Can you work these out from the drawing? Everything is in mm from the part's minimum corner. A direction names the side the tool comes from. Coordinates: 2 decimals unless noted, no trailing zeros. Loops run counter-clockwise (first coordinate to the right, second up) from the corner with the lowest first, then second, coordinate; pieces in that order, holes last. Notation, with made-up numbers: (50.25, -39.75) -> (95.25, -39.75) arc R25 ccw to (95.25, -25.75) -> close; hole circle Ø6 at (-18, -26.5). An arc over 180 degrees is marked (long way). One line per question, with ' | ' between items.
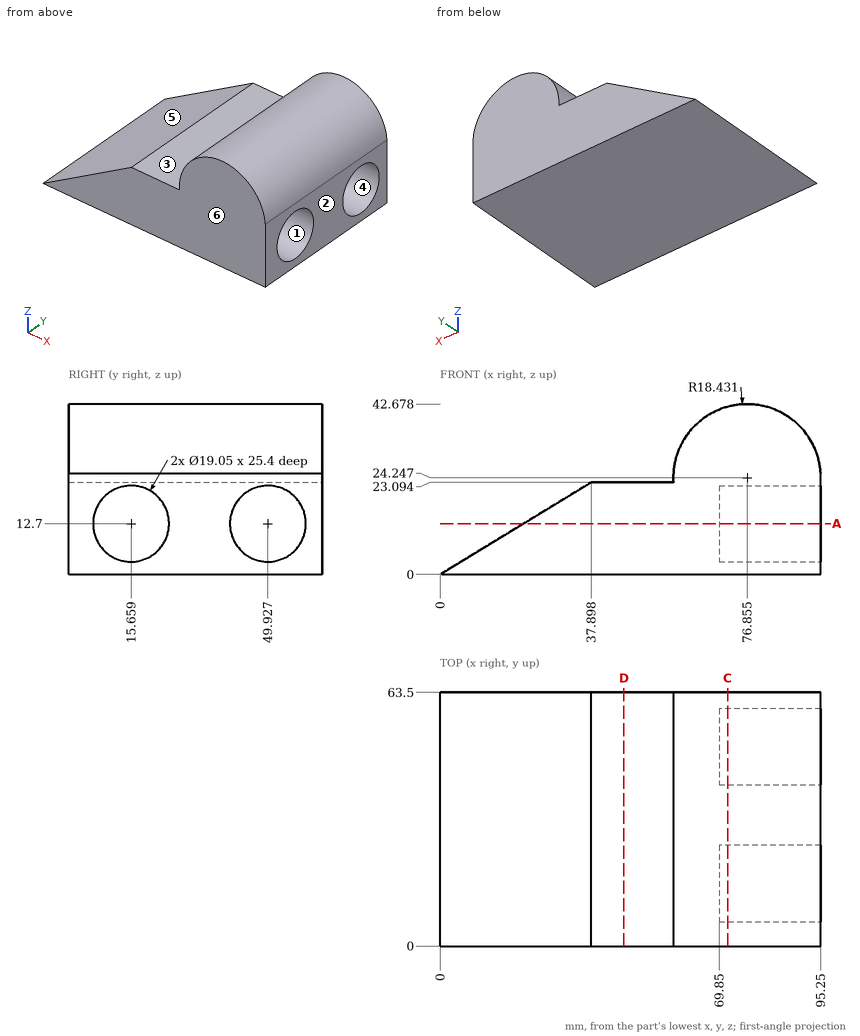
Q1. Please list where these lines run through material, in increasing order: L1, parallel to Y at x = 86, z = 12; L2, parallel to Z at x = 52, y = 34.5 (1 decimal); L3, parallel to Z at x = 71.5, y = 48 (1 decimal). Write a range as [from, to].
Values follow:
L1: y = [0, 6.16], [25.16, 40.43], [59.43, 63.5] | L2: z = [0, 23.1] | L3: z = [0, 3.4], [22, 41.9]
Q2. We'd pull the mould along Y, two halves only. Please class the marked faces 4, 5 and 6: released by +Y, released by -Y, zero draft, split by the parting line, or undercut.
Values follow:
face 4: undercut | face 5: zero draft | face 6: released by -Y
Q3. Imagine slicing it at C-C on x = 72. Give the number of separate pieces and of enclosed holes in the cut face, plus the area to 3 significant figures.
Values follow:
separate pieces: 1 | enclosed holes: 2 | area: 2,100 mm2
Q4. Imagine slicing it at D-D on x = 46. Write out the boundary of the cut face in (y, z) (1 decimal).
Values follow:
outline: (0, 0) -> (63.5, 0) -> (63.5, 23.1) -> (0, 23.1) -> close
Q5. Imagine slicing it at A-A on z = 12.7. Write out the boundary of the cut face in (x, y), plus the area to 3 significant figures.
Values follow:
outline: (20.84, 0) -> (95.25, 0) -> (95.25, 6.13) -> (69.85, 6.13) -> (69.85, 25.18) -> (95.25, 25.18) -> (95.25, 40.4) -> (69.85, 40.4) -> (69.85, 59.45) -> (95.25, 59.45) -> (95.25, 63.5) -> (20.84, 63.5) -> close | area: 3,760 mm2
Q6. For pin 1 (17 mm diameter, centred on y = 49.93, z = 12.7, fed in from -X) (1 decimal); pin 2 (22.5 mm diameter, centred on x = 50.5, y = 42.5, fed in from +Z); pin 3 (11.5 mm diameter, centred on y = 15.66, z = 12.7, fed in from +X), each with a flat end and sliding along its axis, tell me the tip position at first contact or that it passes through.
Values follow:
pin 1: stops at x = 6.9 | pin 2: stops at z = 34.81 | pin 3: stops at x = 69.85
Q7. For the marked faces 1, 2 and 3, which set-ups out of +Z, -Z, +X, -X, +Y, -Y let a thin tool reach every point of the face, with its end or its side?
Values follow:
face 1: +X | face 2: +Z, -Z, +X, +Y, -Y | face 3: +Z, -X, +Y, -Y
